```python
from build123d import *

# Parameters (mm, degrees)
SKETCH2_R                = 35.5
SKETCH2_R_2              = 12.5
BOSS_EXTRUDE1_DEPTH      = 12.5
SKETCH4_R                = 23
CUT_EXTRUDE1_DEPTH       = 10
SKETCH5_R                = 3
CUT_EXTRUDE2_DEPTH       = 53.397519025
CIRPATTERN1_COUNT        = 5
BOSS_EXTRUDE2_DEPTH      = 2
BOSS_EXTRUDE2_DEPTH_BACK = 7
SKETCH6_R                = 13.5
SKETCH6_R_2              = 12.5


with BuildPart() as part:
    # Sketch2 → Boss-Extrude1 (new, symmetric)
    with BuildSketch(Plane.YZ):
        with Locations(Location((0, 0, 0), (0, 0, 270))):
            Circle(SKETCH2_R)
        with Locations(Location((0, 0, 0), (0, 0, 270))):
            Circle(SKETCH2_R_2, mode=Mode.SUBTRACT)
    extrude(amount=BOSS_EXTRUDE1_DEPTH, both=True)

    # Sketch4 → Cut-Extrude1 (cut)
    with BuildSketch(Plane.YZ.offset(12.5)):
        with Locations(Location((0, 0, 0), (0, 0, 270))):
            Circle(SKETCH4_R)
    cut_extrude1 = extrude(amount=-CUT_EXTRUDE1_DEPTH, mode=Mode.SUBTRACT)

    # Mirror1: Cut-Extrude1 across plane
    add(cut_extrude1.mirror(Plane(origin=(0, 0, 0), x_dir=(0, 0, 1), z_dir=(1, 0, 0))), mode=Mode.SUBTRACT)

    # Sketch5 → Cut-Extrude2 (cut, through all)
    with BuildSketch(Plane.YZ.offset(2.5)):
        with Locations(Location((0, 17, 0), (0, 0, 270))):
            Circle(SKETCH5_R)
    cut_extrude2 = extrude(amount=-CUT_EXTRUDE2_DEPTH, mode=Mode.SUBTRACT)

    # CirPattern1: Cut-Extrude2 ×5 about axis
    cirpattern1_axis = Axis((0, 0, 0), (1, 0, 0))
    for i in range(1, CIRPATTERN1_COUNT):
        add(cut_extrude2.rotate(cirpattern1_axis, i * 360 / CIRPATTERN1_COUNT), mode=Mode.SUBTRACT)

    # Sketch6 → Boss-Extrude2 (add, two sides: drawn at the far end of the back side and taken through both)
    with BuildSketch(Plane.YZ.offset(2.5).offset(-BOSS_EXTRUDE2_DEPTH_BACK)):
        with Locations(Location((0, 0, 0), (0, 0, 270))):
            Circle(SKETCH6_R)
        with Locations(Location((0, 0, 0), (0, 0, 270))):
            Circle(SKETCH6_R_2, mode=Mode.SUBTRACT)
    extrude(amount=BOSS_EXTRUDE2_DEPTH + BOSS_EXTRUDE2_DEPTH_BACK)

    # Sketch7 → Cut-Revolve1 (revolve, cut)
    with BuildSketch(Plane(origin=(0, 0, 0), x_dir=(0, 1, 0), z_dir=(0, 0, 1)), mode=Mode.PRIVATE) as cut_revolve1_sk:
        Polygon((-35.5, 9.5), (-29.5, 6.035898385), (-29.5, -6.035898385), (-35.5, -9.5), align=None)
    revolve(cut_revolve1_sk.sketch.rotate(Axis((0, 0, 0), (-1, 0, 0)), 270), axis=Axis((0, 0, 0), (-1, 0, 0)), mode=Mode.SUBTRACT)


solid = part.part
```
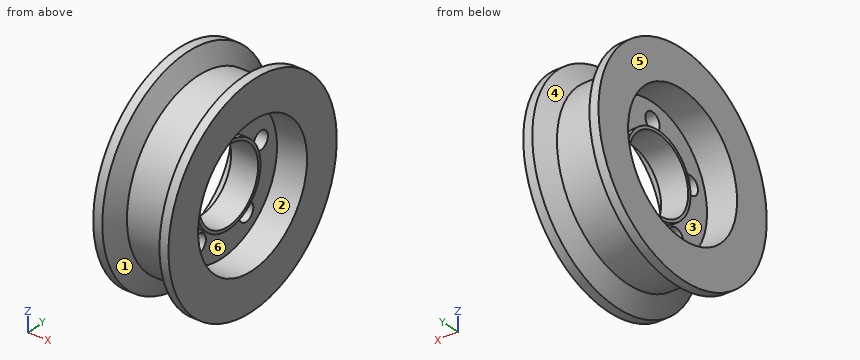
Verification items for the finished model (mm, model axes). Face numbers are marked on the shaded views. A direction names the side the tool comes from. Round coordinates to 2 decimals unless told otherwise and drop trailing zeros. Order: outer loops, then holes, each group sorted by start corner. A loop starts at its lowest first (then second) coordinate and runs counter-clockwise, first axis right, second up. Notation, with made-up numbers: (15, 43) - (54, 43) arc R25 cw to (54, 77) - close; hole circle Ø10 at (-36.5, 45). An arc over 180 degrees is marked (long way). Use CSV: the item, a comma, the result in double quotes. Start each with the question number.
1) Section check B-B, the plane x = 10.5. Record the cut outline in (y, z), plus the area to 3 significant figures.
2) Access from +Z, -Z, +X, -X, +Y, -Y to the whole of each face (thin tool, end or side, straight path). Record for the marked faces 1, 2 and 3.
3) Mould release check, pull along Y, two halves, no side actions. Record for the marked faces 4, 5 and 6: +Y half, -Y half, draft (parallel to the pull), parting line (faces both ways), or undercut.
4) Section check D-D, the plane x = 0.25. Record the cut outline in (y, z).
5) Section check C-C, the plane y = 0. State how many separate pieces and enclosed holes the cut face has, plus the area to 3 significant figures.
6) Go/stop test with flat-tipped pins: P1, Ø3, axis at y = -1.5, z = -16.5, coming from the +X side; P2, Ø1.5, axis at x = 1.5, z = -4, coming from the +Y side; P3, Ø6, axis at y = -28, z = 25, coming from the +X side; P4, Ø3, axis at x = 2.5, z = -8, coming from the +Y side (3 decimals). Record where each tip stops, or that it passes through.
7) Thickness scan on L1, parallel to Z at x = -2.25, y = -11; L2, parallel to Y at x = -0.25, z = -16; L3, parallel to X at y = 17.5, z = 8. Record the ranges inside material, lowest first.
Answers:
1,outline,"circle Ø71 at (0, 0); hole circle Ø46 at (0, 0)"
1,area,"2,300 mm²"
2,face 1,"none"
2,face 2,"+X"
2,face 3,"-X"
3,face 4,"parting line"
3,face 5,"draft"
3,face 6,"undercut"
4,outline,"circle Ø59 at (0, 0); hole circle Ø6 at (-16.17, 5.25); hole circle Ø6 at (-9.99, -13.75); hole circle Ø25 at (0, 0); hole circle Ø6 at (0, 17); hole circle Ø6 at (9.99, -13.75); hole circle Ø6 at (16.17, 5.25)"
5,separate pieces,"3"
5,enclosed holes,"0"
5,area,"522 mm²"
6,P1,"stops at x = 2.5"
6,P2,"stops at y = 29.32"
6,P3,"stops at x = 12.5"
6,P4,"stops at y = 28.775"
7,L1,"z = -27.37 to -16.58, -10.93 to -5.94, 5.94 to 27.37"
7,L2,"y = -24.78 to -11.98, -8 to 8, 11.98 to 24.78"
7,L3,"x = -2.5 to 2.5"
